Source: CAD feature listing. Evaluate the final solid. Frame: model axes, mm. Face numbers are marked on the shaded views. A direction names the side the tool comes from. Round coordinates to 2 decimals unless told otherwise and drop trailing zeros. Write each loop counter-clockwise with the first axis right and the second up, starting at its lowest first coordinate (ties: lowest second). Pieces come first, ordered by that corner, then holes. Notation, with made-up numbers: M 78,42.25 L 89,42.25 A30 cw 89,65.25 Z; hole C -9,46 d2. An arc over 180 degrees is marked long. Use a Markdown table: item, result.
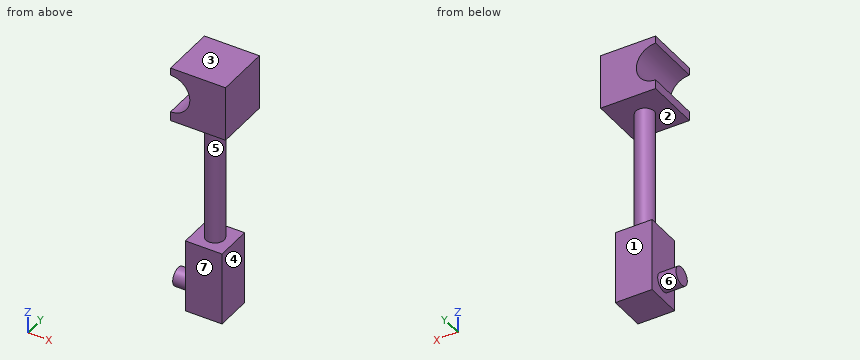
```python
from build123d import *

# Parameters (mm, degrees)
SKETCH1_W           = 20
SKETCH1_H           = 40
BOSS_EXTRUDE1_DEPTH = 20
SKETCH2_R           = 5
BOSS_EXTRUDE2_DEPTH = 10
SKETCH3_R           = 5
BOSS_EXTRUDE3_DEPTH = 70
SKETCH4_W           = 30
SKETCH4_H           = 30
BOSS_EXTRUDE4_DEPTH = 30
CUT_EXTRUDE1_DEPTH  = 30


with BuildPart() as part:
    # Sketch1 → Boss-Extrude1 (new body)
    with BuildSketch(Plane(origin=(0, 0, 0), x_dir=(1, 0, 0), z_dir=(0, 1, 0))):
        with Locations((3.516483516, 1.923076923)):
            Rectangle(SKETCH1_W, SKETCH1_H)
    extrude(amount=BOSS_EXTRUDE1_DEPTH)

    # Sketch2 → Boss-Extrude2 (add)
    with BuildSketch(Plane.ZY.offset(6.483516484)):
        with Locations(Location((-11.923076923, 10, 0), (0, 0, 180))):
            Circle(SKETCH2_R)
    extrude(amount=BOSS_EXTRUDE2_DEPTH)

    # Sketch3 → Boss-Extrude3 (add)
    with BuildSketch(Plane.XY.offset(18.076923077)):
        with Locations((3.516483516, 10)):
            Circle(SKETCH3_R)
    extrude(amount=BOSS_EXTRUDE3_DEPTH)

    # Sketch4 → Boss-Extrude4 (add)
    with BuildSketch(Plane.XY.offset(88.076923077)):
        with Locations((3.516483516, 10)):
            Rectangle(SKETCH4_W, SKETCH4_H)
    extrude(amount=BOSS_EXTRUDE4_DEPTH)

    # Sketch7 → Cut-Extrude1 (cut)
    with BuildSketch(Plane(origin=(0, 25, 0), x_dir=(1, 0, 0), z_dir=(0, 1, 0))):
        with BuildLine():
            ThreePointArc((-11.483516484, -114.035823302), (-1.004066371, -103.55637319), (-11.483516484, -93.076923077))
            Line((-11.483516484, -93.076923077), (-11.483516484, -114.035823302))
        make_face()
    extrude(amount=-CUT_EXTRUDE1_DEPTH, mode=Mode.SUBTRACT)


solid = part.part
```
Q1. Line query: L1, parallel to Z at x = 11, y = 4.5; L2, parallel to Z at x = -6, y = 8; L3, parallel to Z at x = -11, y = 20. Output: solid intervals per line, ascending.
Results are:
| item | result |
|---|---|
| L1 | -21.92 to 18.08, 88.08 to 118.08 |
| L2 | -21.92 to 18.08, 88.08 to 94.63, 112.49 to 118.08 |
| L3 | 88.08 to 93.09, 114.02 to 118.08 |
Q2. Section C-C on z = 23. Return loops of the section in (x, y).
Results are:
| item | result |
|---|---|
| outline | C 3.52,10 d10 |
Q3. Mould query, pull axis Z, two halves, no side actions, for the marked faces 1, 2 and 3. Classes: +Z half, -Z half, draft (parallel to the pull), parting line (faces both ways), or undercut.
Results are:
| item | result |
|---|---|
| face 1 | draft |
| face 2 | undercut |
| face 3 | +Z half |
Q4. Reachability of the marked faces 4, 5, 6 and 7 from +Z, -Z, +X, -X, +Y, -Y: full face, straight path, thin tool, end or side. Return the list, or none.
Results are:
| item | result |
|---|---|
| face 4 | -Z, +X, +Y, -Y |
| face 5 | none |
| face 6 | -X |
| face 7 | -Z, +X, -X, -Y |
Q5. Section B-B on z = -9. Return loops of the section in (x, y).
Results are:
| item | result |
|---|---|
| outline | M -16.48,5.94 L -6.48,5.94 L -6.48,0 L 13.52,0 L 13.52,20 L -6.48,20 L -6.48,14.06 L -16.48,14.06 Z |
Q6. Section D-D on z = 108. Return loops of the section in (x, y).
Results are:
| item | result |
|---|---|
| outline | M -1.99,-5 L 18.52,-5 L 18.52,25 L -1.99,25 Z |
Q7. First-contact query: pin 1 Ø1.2 at (y, z) = (14.5, 116.5) entering from -X; pin 2 Ø6 at (x, z) = (6.5, 2.5) entering from +Y; pin 3 Ø6 at (y, z) = (-1, 3) entering from -X. Flat tips, straight axial feed; report the tip coordinate or a pass-through.
Results are:
| item | result |
|---|---|
| pin 1 | x = -11.48 |
| pin 2 | y = 20 |
| pin 3 | x = -6.48 |
Q8. Section A-A on y = 10. Return loops of the section in (x, z), plus the area to 3 significant figures.
Results are:
| item | result |
|---|---|
| outline | M -16.48,-16.92 L -6.48,-16.92 L -6.48,-21.92 L 13.52,-21.92 L 13.52,18.08 L 8.52,18.08 L 8.52,88.08 L 18.52,88.08 L 18.52,118.08 L -11.48,118.08 L -11.48,114.04 A10.48 cw -11.48,93.08 L -11.48,88.08 L -1.48,88.08 L -1.48,18.08 L -6.48,18.08 L -6.48,-6.92 L -16.48,-6.92 Z |
| area | 2,330 mm^2 |
